The model under review builds one solid part; all positions refer to its coordinate system, in mm. Face numbers are marked on the shaded views. A direction names the side the tool comes from. Coordinates: 2 decimals unless noted, no trailing zeros. Order: outer loops, then holes, each group sorted by start corner. A loop starts at its lowest first (then second) coordinate and runs counter-clockwise, first axis right, second up. Notation, with made-up numbers: M 44,38.25 L 95,38.25 A16 cw 95,53.25 Z; hole C 34.25,34.25 d4. An arc over 180 degrees is marked long. Answer as CSV lines item,"result". Start each with the question number.
Q1. Machinability: for the marked faces 4, 5 and 6, which of the approach directions +Z, -Z, +X, -X, +Y, -Y give a long, thin tool a straight path to every point of the face, cutting with its end or side? Answer none if there is none.
Q2. Consider section A-A on y = 2.35. Write out the cut boundary in (x, z).
Q3. For P1, Ø1.9, axis at y = 2, z = 0, coming from the -X side; P2, Ø0.5, axis at x = 0, y = 2.5, coming from the -Z side; P3, Ø1.2, axis at y = 2, z = -0.5, coming from the +X side, all flat-tipped, find the tip position at first contact; note any pin that passes through.
Q4. The part is to be moulded in two halves that separate along X. For the marked faces 1, 2 and 3, say which applies: +X half, -X half, draft (parallel to the pull), parting line (faces both ways), or undercut.
Q5. Wall thickness on L1, parallel to X at y = 1.2, z = -1; L2, parallel to Z at x = 0.8, y = 2.05; L3, parallel to Y at x = 2.2, z = 2.75: over which ranges is each line inside the solid? List them lowest first. Write a range as [from, to].
Q6. Consider section B-B on z = 0.5. Write out the cut boundary in (x, y), and give its area (3 significant figures).
Q7. Consider section D-D on x = 2.05. Write out the cut boundary in (y, z).
Q8. Consider section C-C on x = -1.8. Write out the cut boundary in (y, z), and give its area (3 significant figures).
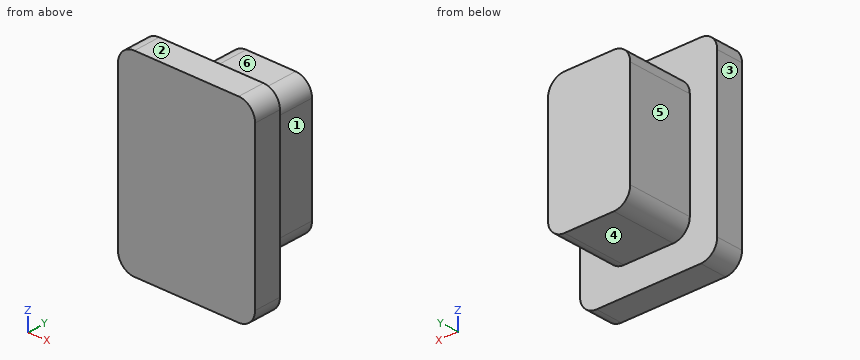
from build123d import *

# Parameters (mm, degrees)
SKETCH_1_W      = 5
SKETCH_1_H      = 7
EXTRUDE_1_DEPTH = 1
SKETCH_2_W      = 3
SKETCH_2_H      = 5
EXTRUDE_2_DEPTH = 2.4
FILLET_1_R      = 0.6


with BuildPart() as part:
    # 草图1 → 凸台-拉伸1 (new body)
    with BuildSketch(Plane(origin=(0, 0, 0), x_dir=(1, 0, 0), z_dir=(0, 1, 0))):
        Rectangle(SKETCH_1_W, SKETCH_1_H)
    extrude(amount=EXTRUDE_1_DEPTH)

    # 草图2 → 凸台-拉伸2 (add)
    with BuildSketch(Plane(origin=(0, 1, 0), x_dir=(1, 0, 0), z_dir=(0, 1, 0))):
        Rectangle(SKETCH_2_W, SKETCH_2_H)
    extrude(amount=EXTRUDE_2_DEPTH)

    # 圆角1
    fillet_1_edges = [part.edges().sort_by_distance(p)[0] for p in [
        (1.5, 2.2, 2.5),
        (1.5, 2.2, -2.5),
        (-1.5, 2.2, -2.5),
        (-1.5, 2.2, 2.5),
        (2.5, 0.5, 3.5),
        (-2.5, 0.5, 3.5),
        (-2.5, 0.5, -3.5),
        (2.5, 0.5, -3.5),
    ]]
    fillet(fillet_1_edges, radius=FILLET_1_R)


solid = part.part
Evaluation:
1,face 4,"-Z, +X, -X, +Y"
1,face 5,"+Z, -Z, -X, +Y"
1,face 6,"+Z, +X, -X, +Y"
2,outline,"M -1.5,-1.9 A0.6 ccw -0.9,-2.5 L 0.9,-2.5 A0.6 ccw 1.5,-1.9 L 1.5,1.9 A0.6 ccw 0.9,2.5 L -0.9,2.5 A0.6 ccw -1.5,1.9 Z"
3,P1,"stops at x = -1.5"
3,P2,"stops at z = -2.5"
3,P3,"stops at x = 1.5"
4,face 1,"+X half"
4,face 2,"draft"
4,face 3,"-X half"
5,L1,"x = [-1.5, 1.5]"
5,L2,"z = [-2.5, 2.5]"
5,L3,"y = [0, 1]"
6,outline,"M -2.5,0 L 2.5,0 L 2.5,1 L 1.5,1 L 1.5,3.4 L -1.5,3.4 L -1.5,1 L -2.5,1 Z"
6,area,"12.2 mm²"
7,outline,"M 0,-3.48 L 1,-3.48 L 1,3.48 L 0,3.48 Z"
8,outline,"M 0,-3.5 L 1,-3.5 L 1,3.5 L 0,3.5 Z"
8,area,"7.00 mm²"
